Geometry check sheet. Reference: the model listing, model coordinates, mm. A direction names the side the tool comes from. Round coordinates to 2 decimals unless told otherwise and drop trailing zeros. Write each loop counter-clockwise with the first axis right and the second up, starting at its lowest first coordinate (ties: lowest second). Pieces come first, ordered by that corner, then holes. Notation, with made-up numbers: (57.5, 16.5) - (86.5, 16.5) arc R18 cw to (86.5, 23.5) - close; hole circle Ø2 at (27.25, 34.25). An arc over 180 degrees is marked (long way). Return JSON: item names as keys, results as strings.
```python
from build123d import *

# Parameters (mm, degrees)
SKETCH1_R           = 22.5
BOSS_EXTRUDE1_DEPTH = 10
BOSS_EXTRUDE2_DEPTH = 20
SKETCH3_R           = 16.5
CUT_EXTRUDE2_DEPTH  = 5


with BuildPart() as part:
    # Sketch1 → Boss-Extrude1 (new body)
    with BuildSketch(Plane(origin=(0, 0, 0), x_dir=(1, 0, 0), z_dir=(0, 1, 0))):
        with Locations(Location((0, 0, 0), (0, 0, 270))):
            Circle(SKETCH1_R)
    extrude(amount=BOSS_EXTRUDE1_DEPTH)

    # Sketch2 → Boss-Extrude2 (add)
    with BuildSketch(Plane(origin=(0, 10, 0), x_dir=(1, 0, 0), z_dir=(0, 1, 0))):
        Polygon((-13.806150904, 27.316911445), (14.687438839, 27.316911445), (14.687438839, 17.819048198), (5.189575591, 17.819048198), (5.189575591, -25.599755221), (-4.308287657, -25.599755221), (-4.308287657, 17.819048198), (-13.806150904, 17.819048198), align=None)
    extrude(amount=BOSS_EXTRUDE2_DEPTH)

    # Sketch3 → Cut-Extrude2 (cut)
    with BuildSketch(Plane.XZ):
        with BuildLine():
            ThreePointArc((-14.551420086, 2.778571429), (0, 11.5), (14.551420086, 2.778571429))
            Line((14.551420086, 2.778571429), (4.83856504, 20.948467447))
            ThreePointArc((4.83856504, 20.948467447), (0, 21.5), (-4.83856504, 20.948467447))
            Line((-4.83856504, 20.948467447), (-14.551420086, 2.778571429))
        make_face()
        with Locations((0, -5)):
            Circle(SKETCH3_R)
    extrude(amount=-CUT_EXTRUDE2_DEPTH, mode=Mode.SUBTRACT)


solid = part.part
```
(1) Section check A-A, the plane y = 21. Enter the section's corners in (x, z).
Response values:
{"outline": "(-13.81, -27.32) - (14.69, -27.32) - (14.69, -17.82) - (5.19, -17.82) - (5.19, 25.6) - (-4.31, 25.6) - (-4.31, -17.82) - (-13.81, -17.82) - close"}
(2) Section check D-D, the plane y = 3.5. Enter the section's corners in (x, z).
Response values:
{"outline": "circle Ø45 at (0, 0); hole (-14.55, 2.78) arc R16.5 ccw (long way) to (14.55, 2.78) - (4.84, 20.95) arc R21.5 ccw to (-4.84, 20.95) - close"}
(3) Gauge pin test, flat ends, axial feed: pin 1 (3 mm diameter, centred on y = 21.5, z = 15.5, fed in from +X); pin 2 (9 mm diameter, centred on x = -15, z = 4, fed in from +Y); pin 3 (7.5 mm diameter, centred on x = -11, y = 15.5, fed in from +Z); pin 4 (7.5 mm diameter, centred on x = 5, z = -24.5, fed in from -Y). Record the tip position at first contact, or that the pin passes through.
Response values:
{"pin 1": "stops at x = 5.19", "pin 2": "stops at y = 10", "pin 3": "stops at z = -17.82", "pin 4": "stops at y = 0"}
(4) Section check B-B, the plane x = 0. Enter the section's corners in (y, z), plus the area to 3 significant figures.
Response values:
{"outline": "(0, -22.5) - (10, -22.5) - (10, -27.32) - (30, -27.32) - (30, 25.6) - (10, 25.6) - (10, 22.5) - (0, 22.5) - (0, 21.5) - (5, 21.5) - (5, -21.5) - (0, -21.5) - close", "area": "1,290 mm^2"}
(5) Section check C-C, the plane z = -14.5. Enter the section's corners in (x, y), plus the area to 3 significant figures.
Response values:
{"outline": "(-17.2, 0) - (-13.49, 0) - (-13.49, 5) - (13.49, 5) - (13.49, 0) - (17.2, 0) - (17.2, 10) - (5.19, 10) - (5.19, 30) - (-4.31, 30) - (-4.31, 10) - (-17.2, 10) - close", "area": "399 mm^2"}
(6) Release check for a two-part mould opening along X. For faces 1 (the face through (-0.476, 2.465, -21.493)), 2 (the face through (-8.618, 4.93, 20.784)), 3 (the face through (0.1, 2.5, 21.5)), 4 (the face through (1, 20, 25.6)) record: pulls with the +X half, pulls with the -X half, needs draft (parallel to the pull), parting line crosses it, or undercut.
Response values:
{"face 1": "undercut", "face 2": "parting line crosses it", "face 3": "undercut", "face 4": "needs draft"}
(7) Access from +Z, -Z, +X, -X, +Y, -Y to the whole of each face (thin tool, end or side, straight path). Record for faces 5 (the face through (12, 0, 8)), 6 (the face through (12, 10, 2)), 7 (the face through (0, 20, -27.317)), 8 (the face through (-4.308, 20, 4)), 9 (the face through (9.76, 2.46, 11.74)).
Response values:
{"face 5": "+Z, -Z, +X, -X, -Y", "face 6": "+Z, +X, +Y", "face 7": "-Z, +X, -X, +Y, -Y", "face 8": "+Z, -X, +Y", "face 9": "-Y"}
(8) Material ranges on line 1 along Z through (x, y) = (12.5, 11.25); line 2 along Y through (x, z) = (-14.5, 14); line 3 along X through (y, z) = (23, -15.5), recorded low to high. Write a range as [from, to].
Response values:
{"line 1": "z = [-27.32, -17.82]", "line 2": "y = [0, 10]", "line 3": "x = [-4.31, 5.19]"}
